Part model, mm, in its own coordinate system. Face numbers are marked on the shaded views. A direction names the side the tool comes from. Give positions to 0.01 mm unless a question says otherwise; leave off trailing zeros. Write each loop counter-clockwise with the first axis right and the second up, starting at its lowest first coordinate (ties: lowest second). Pieces come first, ordered by that corner, then holes. Notation, with made-up numbers: (-4, -19.5) - (1, -19.5) arc R15 ccw to (1, -5.5) - close; hole circle Ø5 at (19.25, 49). An arc over 180 degrees is marked (long way). Answer in a Markdown table with one row per item. Add a question column.
1. Band-saw the part on A-A on z = -11. Write the cut outline in (x, y), plus the area to 3 significant figures.
2. Band-saw the part on C-C on x = 9. Write the cut outline in (y, z), plus the area to 3 significant figures.
3. Drop flat-ended pins along their axis: pin 1 Ø3 at (x, z) = (-18, -5.5) entering from +Y; pin 2 Ø0.8 at (x, y) = (-19, 3) entering from -Z; pin 3 Ø4 at (x, y) = (-0.5, 21.5) entering from -Z. Give the stop position or say it passes through.
4. Which spindle directions (+Z, -Z, +X, -X, +Y, -Y) get a long thin tool onto all of the face, cutting with end or side? Do the marked faces 1, 2, 3 and 4. Say none if no direction does.
5. Probe line 1 along Z through (x, y) = (16.5, 8); line 2 along X through (y, z) = (22, 1.55); line 3 along X through (y, z) = (22.25, 0.75). List the from-to ranges inside material, lowest first.
6. Band-saw the part on B-B on y = 17.5. Write the cut outline in (x, z).
7. Band-saw the part on D-D on y = 22. Write the cut outline in (x, z).
8. Pull direction X, two halves, no side cores. Call the marked faces 5, 6 and 7: released by +X, released by -X, zero draft, split by the parting line, or undercut.
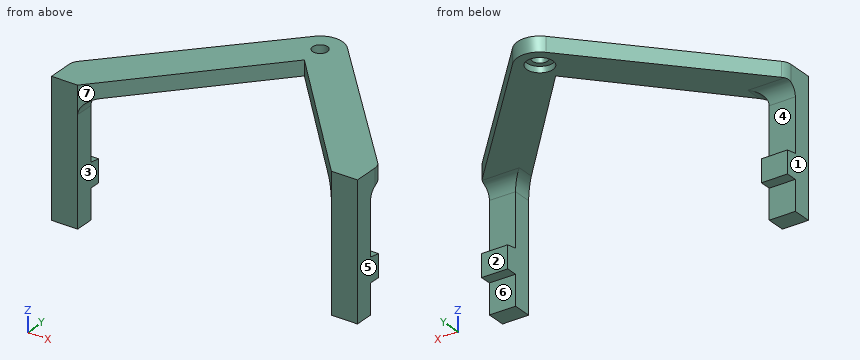
```python
from build123d import *

# Parameters (mm, degrees)
F0_W           = 3.5
F0_H           = 4
F1_DEPTH       = 2
F2_D           = 2
F2_CBORE_D     = 3.5
F2_CBORE_DEPTH = 0.8
F3_DEPTH       = 12
F5_DEPTH       = 41.001
F6_R           = 1.6899494937
F7_W           = 3.5
F7_H           = 2.5
F8_DEPTH       = 4


with BuildPart() as f1:
    # F0 (on Top) → F1 (new body)
    with BuildSketch(Plane.XY):
        with BuildLine():
            Line((-17, 0), (0, 19))
            ThreePointArc((0, 19), (-2.7448989049, 20.7894092344), (-2.2152995112, 24.0229799988))
            Line((-2.2152995112, 24.0229799988), (-20.5, 4))
            Line((-20.5, 4), (-17, 4))
            Line((-17, 4), (-17, 0))
        make_face()
        with BuildLine():
            ThreePointArc((0, 19), (2.1213203436, 19.8786796564), (3, 22))
            ThreePointArc((3, 22), (2.7969535689, 23.0849196898), (2.2152995112, 24.0229799988))
            ThreePointArc((2.2152995112, 24.0229799988), (0, 25), (-2.2152995112, 24.0229799988))
            ThreePointArc((-2.2152995112, 24.0229799988), (-2.7448989049, 20.7894092344), (0, 19))
        make_face()
        with BuildLine():
            ThreePointArc((2.2152995112, 24.0229799988), (2.7969535689, 23.0849196898), (3, 22))
            ThreePointArc((3, 22), (2.1213203436, 19.8786796564), (0, 19))
            Line((0, 19), (17, 0))
            Line((17, 0), (17, 4))
            Line((17, 4), (20.5, 4))
            Line((20.5, 4), (2.2152995112, 24.0229799988))
        make_face()
        with Locations((-18.75, 2)):
            Rectangle(F0_W, F0_H)
        with Locations((18.75, 2)):
            Rectangle(F0_W, F0_H)
    extrude(amount=F1_DEPTH)

    # F2 (through all)
    with Locations(Plane(origin=(0, 0, 0), x_dir=(1, 0, 0), z_dir=(0, 0, -1))):
        with Locations((0, -22)):
            CounterBoreHole(F2_D / 2, F2_CBORE_D / 2, F2_CBORE_DEPTH)

    # F0 (on Top) → F3 (join)
    with BuildSketch(Plane.XY):
        with Locations((18.75, 2)):
            Rectangle(F0_W, F0_H)
        with Locations((-18.75, 2)):
            Rectangle(F0_W, F0_H)
    extrude(amount=-F3_DEPTH)

    # F4 (on face) → F5 (cut, through all)
    with BuildSketch(Plane.YZ.offset(20.5)):
        Polygon((4, -9), (4, 0), (2.5, 0), (2.5, -8.75), align=None)
    extrude(amount=-F5_DEPTH, mode=Mode.SUBTRACT)

    # F6 (call 1 of 4: OpenCascade refuses the feature's edges together)
    f6_edges = [f1.edges().sort_by_distance(p)[0] for p in [
        (20.5, 4, 1),
    ]]
    fillet(f6_edges, radius=F6_R)

    # F6#2 (call 2 of 4)
    f6_2_edges = [f1.edges().sort_by_distance(p)[0] for p in [
        (-20.5, 4, 1),
    ]]
    fillet(f6_2_edges, radius=F6_R)

    # F6#3 (call 3 of 4)
    f6_3_edges = [f1.edges().sort_by_distance(p)[0] for p in [
        (-17, 1.25, 0),
        (-18.75, 2.5, 0),
    ]]
    fillet(f6_3_edges, radius=F6_R)

    # F6#4 (call 4 of 4)
    f6_4_edges = [f1.edges().sort_by_distance(p)[0] for p in [
        (18.75, 2.5, 0),
        (17, 1.25, 0),
    ]]
    fillet(f6_4_edges, radius=F6_R)

    # F7 (on face) → F8 (join)
    with BuildSketch(Plane(origin=(0, 0, -12), x_dir=(1, 0, 0), z_dir=(0, 0, -1))):
        with Locations((18.75, -1.25)):
            Rectangle(F7_W, F7_H)
        with Locations((-18.75, -1.25)):
            Rectangle(F7_W, F7_H)
    extrude(amount=F8_DEPTH)


solid = f1.part
```
Values:
| question | item | result |
|---|---|---|
| 1 | outline | (-20.5, 0) - (-17, 0) - (-17, 4) - (-20.5, 4) - close; (17, 0) - (20.5, 0) - (20.5, 4) - (17, 4) - close |
| 1 | area | 28.0 mm² |
| 2 | outline | (8.94, 0) - (16.59, 0) - (16.59, 2) - (8.94, 2) - close |
| 2 | area | 15.3 mm² |
| 3 | pin 1 | stops at y = 2.5 |
| 3 | pin 2 | stops at z = -12 |
| 3 | pin 3 | stops at z = 0 |
| 4 | face 1 | +Z, -Z, -X, +Y, -Y |
| 4 | face 2 | -Z, +X, -X, +Y |
| 4 | face 3 | -Z, +Y, -Y |
| 4 | face 4 | +X, -X, +Y |
| 5 | line 1 | z = 0 to 2 |
| 5 | line 2 | x = -4.06 to -1, 1 to 4.06 |
| 5 | line 3 | x = -3.83 to -1.73, 1.73 to 3.83 |
| 6 | outline | (-8.17, 0) - (-1.34, 0) - (-1.34, 2) - (-8.17, 2) - close; (1.34, 0) - (8.17, 0) - (8.17, 2) - (1.34, 2) - close |
| 7 | outline | (-4.06, 0) - (-1.75, 0) - (-1.75, 0.8) - (-1, 0.8) - (-1, 2) - (-4.06, 2) - close; (1, 0.8) - (1.75, 0.8) - (1.75, 0) - (4.06, 0) - (4.06, 2) - (1, 2) - close |
| 8 | face 5 | released by +X |
| 8 | face 6 | zero draft |
| 8 | face 7 | undercut |
